Part model, mm, in its own coordinate system. Coordinates: 2 decimals unless noted, no trailing zeros. Loops run counter-clockwise (first coordinate to the right, second up) from the corner with the lowest first, then second, coordinate; pieces in that order, holes last. Notation, with made-up numbers: (40, 16) -> (97, 16) arc R18 cw to (97, 34) -> close; hole circle Ø4 at (-19.75, 66). An arc over 180 degrees is marked (long way). One line per item, written item: value. Start each with the question number.
from build123d import *

# Parameters (mm, degrees)
REVOLVE1_ANGLE     = 180
SKETCH2_W          = 3
SKETCH2_H          = 3
CUT_EXTRUDE1_DEPTH = 6


with BuildPart() as part:
    # Sketch1 → Revolve1 (revolve)
    with BuildSketch(Plane(origin=(0, 76.75, 0), x_dir=(-1, 0, 0), z_dir=(0, -1, 0))):
        with BuildLine():
            Line((-13.5, -0.25), (7, -0.25))
            ThreePointArc((7, -0.25), (-3.25, -10.5), (-13.5, -0.25))
        make_face()
    revolve(axis=Axis((13.5, 76.75, 0.25), (-1, 0, 0)), revolution_arc=REVOLVE1_ANGLE)

    # Sketch2 → Cut-Extrude1 (cut)
    with BuildSketch(Plane.XZ.offset(-76.75)):
        with Locations((3.25, 0.25)):
            Rectangle(SKETCH2_W, SKETCH2_H)
    extrude(amount=-CUT_EXTRUDE1_DEPTH, mode=Mode.SUBTRACT)


solid = part.part
1) Pull direction X, two halves, no side cores. Call faces 1 (the flat face through (3, 76.75, 2)), 2 (the flat face through (3, 80, 1.75)): +X half, -X half, draft (parallel to the pull), parting line (faces both ways), or undercut.
2) Pin check, flat tips, straight feed: pin 1 Ø3.5 at (y, z) = (79, 0) entering from -X; pin 2 Ø1.5 at (y, z) = (79, 3.5) entering from -X; pin 3 Ø1.5 at (x, y) = (3, 80.5) entering from -Z. Stop position of each tip, or through.
3) Slice it at B-B (x = 4). Give the cut face in (y, z), then the cut area to 3 significant figures.
4) Slice it at D-D (y = 78). Give the cut face in (x, z), then the cut area to 3 significant figures.
5) Slice it at A-A (y = 80.5). Give the cut face in (x, z), then the cut area to 3 significant figures.
6) Slice it at C-C (z = -0.25). Give the cut face in (x, y), then the cut area to 3 significant figures.
7) Probe line 1 (Z direction, x = 3.5, y = 81); line 2 (Z direction, x = 3, y = 79.75); line 3 (Z direction, x = -4, y = 81.5). List the from-to ranges inside material, lowest first. Write a range as from..to.
Check sheet entries:
1. face 1: draft
1. face 2: undercut
2. pin 1: stops at x = -6.99
2. pin 2: stops at x = -6.49
2. pin 3: stops at z = -9.55
3. outline: (76.75, -9.97) arc R10.22 ccw to (76.75, 10.47) -> (76.75, 1.75) -> (82.75, 1.75) -> (82.75, -1.25) -> (76.75, -1.25) -> close
3. area: 146 mm^2
4. outline: circle Ø20.35 at (3.25, 0.25); hole (1.75, -1.25) -> (4.75, -1.25) -> (4.75, 1.75) -> (1.75, 1.75) -> close
4. area: 316 mm^2
5. outline: circle Ø19.08 at (3.25, 0.25); hole (1.75, -1.25) -> (4.75, -1.25) -> (4.75, 1.75) -> (1.75, 1.75) -> close
5. area: 277 mm^2
6. outline: (-6.99, 76.75) -> (1.75, 76.75) -> (1.75, 82.75) -> (4.75, 82.75) -> (4.75, 76.75) -> (13.49, 76.75) arc R10.24 ccw to start
6. area: 147 mm^2
7. line 1: z = -9.07..-1.25, 1.75..9.57
7. line 2: z = -9.55..-1.25, 1.75..10.05
7. line 3: z = -5.22..5.72
